Part print with two shaded views. Sizes in mm from the minimum x, y, z corner. A direction names the side the tool comes from. Give positions to 0.01 mm unless a question says otherwise; leave off trailing zeros. Write each loop counter-clockwise with the first axis right and the second up, starting at its lowest first coordinate (ties: lowest second). Pieces come first, ordered by that corner, then holes. Notation, with made-up numbers: (-6, 35.5) - (14, 35.5) arc R28 ccw to (14, 71.5) - close; hole circle Ø6 at (-15, 64). An arc over 180 degrees is marked (long way). One line per item, written item: value. Start each with the question number.
(1) Probe L1, parallel to X at y = 25.75, z = 57.5; L2, parallel to Z at x = 8.5, y = 11; L3, parallel to Y at x = 154.5, z = 27. List the from-to ranges inside material, lowest first.
(2) Drop flat-ended pins along their axis: P1, Ø2, axis at x = 33.5, y = 18, coming from the -Z side; P2, Ø1.5, axis at x = 30, z = 25, coming from the +Y side. Give the stop position or say it passes through.
(3) Cut at A-A, the plane x = 150. List the corners of the cut face in (y, z).
(4) Cut at C-C, the plane z = 37. List the corners of the cut face in (x, y).
(5) Mould opens along Z. For the marked faces 3, 4 and 5 say: pulls with the +Z half, pulls with the -Z half, needs draft (parallel to the pull), parting line crosses it, or undercut.
(6) Cut at B-B, the plane y = 8.5. List the corners of the cut face in (x, z), and give its area (3 significant figures).
(7) 3-axis set-ups, long thin cutter, end or side, ignore diameter. For the marked faces 1 and 2: which of +Z, -Z, +X, -X, +Y, -Y reach the whole face in a straight line?
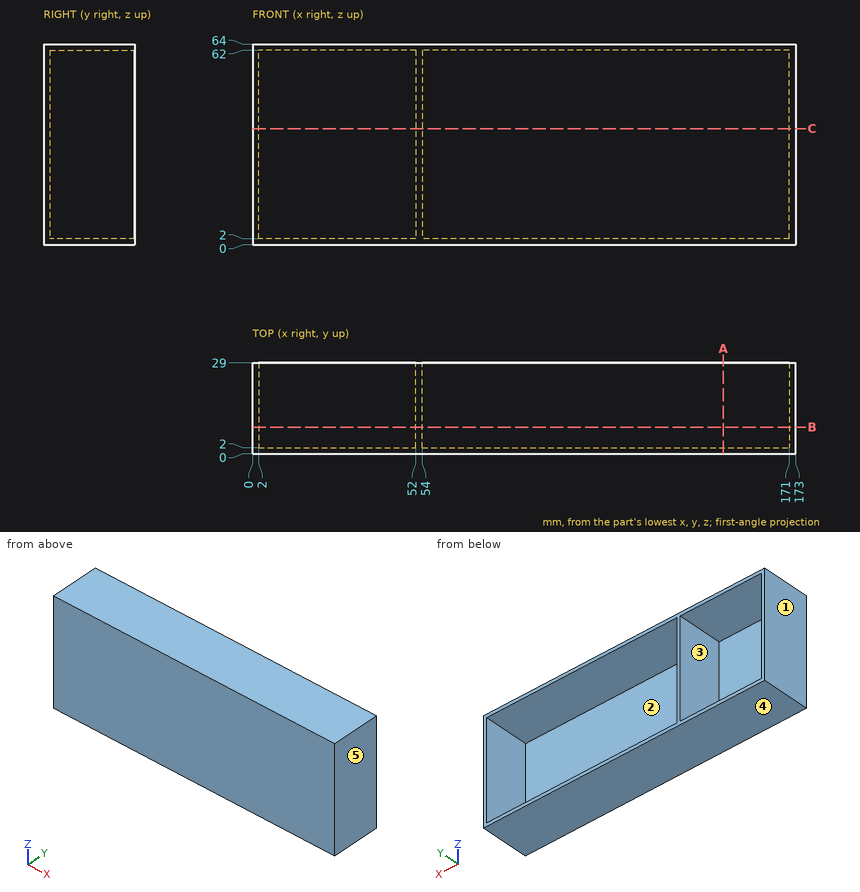
Answers follow:
1. L1: x = 0 to 2, 52 to 54, 171 to 173
1. L2: z = 0 to 2, 62 to 64
1. L3: y = 0 to 2
2. P1: stops at z = 0
2. P2: stops at y = 2
3. outline: (0, 0) - (29, 0) - (29, 2) - (2, 2) - (2, 62) - (29, 62) - (29, 64) - (0, 64) - close
4. outline: (0, 0) - (173, 0) - (173, 29) - (171, 29) - (171, 2) - (54, 2) - (54, 29) - (52, 29) - (52, 2) - (2, 2) - (2, 29) - (0, 29) - close
5. face 3: undercut
5. face 4: pulls with the -Z half
5. face 5: needs draft
6. outline: (0, 0) - (173, 0) - (173, 64) - (0, 64) - close; hole (2, 2) - (52, 2) - (52, 62) - (2, 62) - close; hole (54, 2) - (171, 2) - (171, 62) - (54, 62) - close
6. area: 1,050 mm²
7. face 1: +Z, -Z, -X, +Y, -Y
7. face 2: +Y
